Source: CAD feature listing. Evaluate the final solid. Frame: model axes, mm. A direction names the side the tool comes from. Coordinates: 2 decimals unless noted, no trailing zeros. Write each loop counter-clockwise with the first axis right and the second up, starting at its lowest first coordinate (ties: lowest second). Pieces come first, ordered by that corner, then holes. Notation, with made-up numbers: M 57,-30.75 L 78,-30.75 A16 cw 78,-6.75 Z; hole C 83.25,17 d10. An arc over 180 degrees is marked long. Write item = value, one per line. Start each with the question number.
1. Pin query (flat end, axial travel): pin 1 Ø2 at (y, z) = (60.5, -11) entering from +X; pin 2 Ø9.5 at (y, z) = (30, 7.5) entering from +X; pin 3 Ø5 at (y, z) = (5.5, 12.5) entering from -X. Return the tip coordinate at first contact, or that it passes through.
2. Access query for faces 4 (the face through (0, 63, 1)), 5 (the face through (0, 66, 1)), 6 (the face through (1, 34, -17.5)). Directions: +Z, -Z, +X, -X, +Y, -Y. A direction counts if a zero-diameter tool reaches every point of the face in a straight line with its end or side. Return the directions, or none.
3. Section query A-A (y = 42). Output: boundary loops of the cut face in (x, z), then the cut area to 3 significant figures.
4. Section query B-B (x = 0.5). Output: boundary loops of the cut face in (y, z).
5. Line query: line 1 along X through (y, z) = (65.5, -0.5); line 2 along X through (y, z) = (62, 6); line 3 along Z through (x, y) = (45, -1.7). Output: solid intervals per line, ascending.
6. Section query C-C (z = 15). Output: boundary loops of the cut face in (x, y).
7. Section query D-D (x = -52). Output: boundary loops of the cut face in (y, z).
8. Pull-direction query (X, two-part tool) for faces 1 (the face through (-1, 0, -15)), 2 (the face through (-59.34, 33.5, -14.65)), 3 (the face through (64, 34, 0)); classes: pulls with the +X half, pulls with the -X half, needs draft (parallel to the pull), parting line crosses it, or undercut.
```python
from build123d import *

# Parameters (mm, degrees)
F0_R           = 5
F1_DEPTH       = 3
F2_W           = 66
F2_H           = 3
F3_DEPTH       = 66
F4_W           = 60
F4_H           = 60
F5_DEPTH       = 25
F6_R           = 2.5
F7_DEPTH       = 5.9
F8_R           = 1.5
F9_W           = 90
F9_H           = 3
F10_DEPTH      = 69
F10_DEPTH_BACK = 3
F11_W          = 66
F11_H          = 3
F12_DEPTH      = 29
F13_W          = 3
F13_H          = 63
F14_DEPTH      = 29


with BuildPart() as f1:
    # F0 (on Front) → F1 (new body)
    with BuildSketch(Plane.XZ):
        with BuildLine():
            ThreePointArc((45, -17.5), (62.5, 0), (45, 17.5))
            Line((45, 17.5), (-45, 17.5))
            ThreePointArc((-45, 17.5), (-62.5, 0), (-45, -17.5))
            Line((-45, -17.5), (45, -17.5))
        make_face()
        with Locations((45, 0)):
            Circle(F0_R, mode=Mode.SUBTRACT)
    extrude(amount=F1_DEPTH)

    # F2 (on face) → F3 (join)
    with BuildSketch(Plane(origin=(0, 0, 0), x_dir=(-1, 0, 0), z_dir=(0, 1, 0))):
        with Locations((0, -13)):
            Rectangle(F2_W, F2_H)
    extrude(amount=F3_DEPTH)

    # F4 (on face) → F5 (cut)
    with BuildSketch(Plane(origin=(0, 0, -14.5), x_dir=(1, 0, 0), z_dir=(0, 0, -1))):
        with Locations((0, -33)):
            Rectangle(F4_W, F4_H)
    extrude(amount=-F5_DEPTH, mode=Mode.SUBTRACT)

    # F6 (on face) → F7 (join)
    with BuildSketch(Plane(origin=(0, 0, 0), x_dir=(-1, 0, 0), z_dir=(0, 1, 0))):
        with Locations((45, 0)):
            Circle(F6_R)
    extrude(amount=F7_DEPTH)

    # F8
    f8_edges = [f1.edges().sort_by_distance(p)[0] for p in [
        (-42.5, 5.9, 0),
    ]]
    fillet(f8_edges, radius=F8_R)

    # F9 (on face) → F10 (join, two sides)
    with BuildSketch(Plane(origin=(0, 0, 0), x_dir=(-1, 0, 0), z_dir=(0, 1, 0))) as f10_sk:
        with BuildLine():
            Line((65.5, 0), (62.5, 0))
            ThreePointArc((62.5, 0), (57.374369, -12.374369), (45, -17.5))
            Line((45, -17.5), (45, -20.5))
            ThreePointArc((45, -20.5), (59.495689, -14.495689), (65.5, 0))
        make_face()
        with Locations((0, -19)):
            Rectangle(F9_W, F9_H)
        with BuildLine():
            Line((-45, -20.5), (-45, -17.5))
            ThreePointArc((-45, -17.5), (-57.374369, -12.374369), (-62.5, 0))
            Line((-62.5, 0), (-65.5, 0))
            ThreePointArc((-65.5, 0), (-59.495689, -14.495689), (-45, -20.5))
        make_face()
    extrude(amount=F10_DEPTH)
    extrude(f10_sk.sketch, amount=-F10_DEPTH_BACK)

    # F11 (on face) → F12 (join)
    with BuildSketch(Plane.XY.offset(-11.5)):
        with Locations((0, 64.5)):
            Rectangle(F11_W, F11_H)
    extrude(amount=F12_DEPTH)

    # F13 (on face) → F14 (join)
    with BuildSketch(Plane.XY.offset(-11.5)):
        with Locations((-31.5, 31.5)):
            Rectangle(F13_W, F13_H)
        with Locations((31.5, 31.5)):
            Rectangle(F13_W, F13_H)
    extrude(amount=F14_DEPTH)


solid = f1.part
```
Results are:
q1.pin_1 = 62.9
q1.pin_2 = 33
q1.pin_3 = -33
q2.face_4 = +Z
q2.face_5 = +Z, +Y
q2.face_6 = +Y
q3.outline = M -65.5,0 A20.5 ccw -45,-20.5 L 45,-20.5 A20.5 ccw 65.5,0 L 62.5,0 A17.5 cw 45,-17.5 L -45,-17.5 A17.5 cw -62.5,0 Z; M -33,-14.5 L -30,-14.5 L -30,17.5 L -33,17.5 Z; M 30,-14.5 L 33,-14.5 L 33,17.5 L 30,17.5 Z
q3.area = 641 mm^2
q4.outline = M -3,-20.5 L 69,-20.5 L 69,-17.5 L 0,-17.5 L 0,-14.5 L 3,-14.5 L 3,-11.5 L 0,-11.5 L 0,17.5 L -3,17.5 Z; M 63,-14.5 L 66,-14.5 L 66,17.5 L 63,17.5 Z
q5.line_1 = -65.49 to -62.49, -33 to 33, 62.49 to 65.49
q5.line_2 = -33 to -30, 30 to 33
q5.line_3 = -20.5 to -5, 5 to 17.5
q6.outline = M -54.01,-3 L 54.01,-3 L 54.01,0 L 33,0 L 33,66 L -33,66 L -33,0 L -54.01,0 Z; hole M -30,0 L 30,0 L 30,63 L -30,63 Z
q7.outline = M -3,-19.27 L 69,-19.27 L 69,-16.04 L 0,-16.04 L 0,16.04 L -3,16.04 Z
q8.face_1 = undercut
q8.face_2 = pulls with the -X half
q8.face_3 = needs draft
